Read the model definition and answer for the solid it produces. Units are mm, in the model's axes. Give positions to 0.01 mm unless a question says otherwise; leave off trailing zeros. Write each loop counter-clockwise with the first axis right and the second up, starting at its lowest first coordinate (ties: lowest second). Pieces come first, ordered by that corner, then holes. Notation, with made-up numbers: M -19.75,88.25 L 11.25,88.25 A30 cw 11.25,120.25 Z; hole C 9.5,67 d3. An arc over 180 degrees is marked long. Put each result on its own line as item: value.
Autodesk Inventor part; units mm, degrees
ref_plane "YZ Plane" through (0, 0, 0) normal (1, 0, 0) x (0, 1, 0)
ref_plane "XZ Plane" through (0, 0, 0) normal (0, 1, 0) x (-1, 0, 0)
ref_plane "XY Plane" through (0, 0, 0) normal (0, 0, 1) x (1, 0, 0)
sketch "Sketch1" plane through (0, 0, 0) normal (0, 0, 1) x (1, 0, 0)
  line L0 (-28.6, -15.9) -> (0, -15.9) construction
  line L1 (-28.6, 817.5) -> (-28.6, -17.5) construction
  line L2 (125, 817.5) -> (125, -17.5) construction
  line L3 (96.4, -15.9) -> (125, -15.9) construction
  line L4 (-28.6, 815.9) -> (0, 815.9) construction
  line L5 (96.4, 815.9) -> (125, 815.9) construction
  circle A0 centre (-14.3, 0) radius 2 construction
  circle A1 centre (110.7, 0) radius 2 construction
  circle A2 centre (-14.3, 252.5) radius 2 construction
  circle A3 centre (110.7, 252.5) radius 2 construction
  circle A4 centre (-14.3, 545.5) radius 2 construction
  circle A5 centre (110.7, 545.5) radius 2 construction
  circle A6 centre (-14.3, 800) radius 2 construction
  circle A7 centre (110.7, 800) radius 2 construction
  line L6 (-28.6, -15.9) -> (125, -15.9)
  line L7 (125, -15.9) -> (125, 815.9)
  line L8 (125, 815.9) -> (-28.6, 815.9)
  line L9 (-28.6, 815.9) -> (-28.6, -15.9)
  circle A8 centre (-14.3, 0) radius 4
  circle A9 centre (110.7, 0) radius 4
  circle A10 centre (-14.3, 252.5) radius 4
  circle A11 centre (110.7, 252.5) radius 4
  circle A12 centre (-14.3, 545.5) radius 4
  circle A13 centre (110.7, 545.5) radius 4
  circle A14 centre (-14.3, 800) radius 4
  circle A15 centre (110.7, 800) radius 4
  point P0 (0, 0)
  dimension "d0" = 2
  dimension "d1" = 2
  dimension "d2" = 2
  dimension "d3" = 2
  dimension "d4" = 2
  dimension "d5" = 2
  dimension "d6" = 2
  dimension "d7" = 2
extrude "Extrusion1" add sketch "Sketch1" along normal blind 2
sketch "Sketch2" plane through (0, 0, 2) normal (0, 0, 1) x (1, 0, 0)
  arc A0 (81.2, 144.25) -> (81.2, 152.25) centre (81.2, 148.25) ccw construction
  arc A1 (79.0077, 648.4043) -> (79.0077, 655.0957) centre (81.2, 651.75) ccw construction
  arc A2 (33.1012, 180.4907) -> (33.1012, 116.0093) centre (42.2, 148.25) ccw construction
  arc A3 (33.1012, 683.9907) -> (33.1012, 619.5093) centre (42.2, 651.75) ccw construction
  arc A4 (30.3852, 190.1148) -> (30.3852, 106.3852) centre (42.2, 148.25) ccw
  arc A5 (30.3852, 693.6148) -> (30.3852, 609.8852) centre (42.2, 651.75) ccw
  line L0 (125, -15.9) -> (125, 815.9) construction
  line L1 (30.3852, 106.3852) -> (125, 106.3852)
  line L2 (30.3852, 190.1148) -> (125, 190.1148)
  line L3 (30.3852, 609.8852) -> (125, 609.8852)
  line L4 (30.3852, 693.6148) -> (125, 693.6148)
  line L5 (125, 106.3852) -> (125, 190.1148)
  line L6 (125, 609.8852) -> (125, 693.6148)
  point P0 (0, 0)
  dimension "d10" = 10
  dimension "d11" = 10
  dimension "d16" = 83.7296
  dimension "d17" = 83.7296
  dimension "d18" = 41.8648
  dimension "d19" = 41.8648
extrude "Extrusion2" cut sketch "Sketch2" against normal blind 2
fillet "Fillet1" radius 2 8 edges at (-28.6, -15.9, 1) (125, -15.9, 1) (-28.6, 815.9, 1) (125, 815.9, 1) (125, 693.6148, 1) (125, 609.8852, 1) (125, 106.3852, 1) (125, 190.1148, 1)
sketch "Sketch3" plane through (0, 0, 2) normal (0, 0, 1) x (1, 0, 0)
  arc A0 (123, 190.1148) -> (125, 192.1148) centre (123, 192.1148) ccw construction
  line L0 (125, 192.1148) -> (125, 607.8852) construction
  arc A1 (125, 607.8852) -> (123, 609.8852) centre (123, 607.8852) ccw construction
  line L1 (123, 609.8852) -> (30.3852, 609.8852) construction
  arc A2 (30.3852, 693.6148) -> (30.3852, 609.8852) centre (42.2, 651.75) ccw construction
  line L2 (30.3852, 693.6148) -> (123, 693.6148) construction
  arc A3 (123, 693.6148) -> (125, 695.6148) centre (123, 695.6148) ccw construction
  line L3 (125, 695.6148) -> (125, 813.9) construction
  arc A4 (125, 813.9) -> (123, 815.9) centre (123, 813.9) ccw construction
  line L4 (123, 815.9) -> (-26.6, 815.9) construction
  arc A5 (-26.6, 815.9) -> (-28.6, 813.9) centre (-26.6, 813.9) ccw construction
  line L5 (-28.6, 813.9) -> (-28.6, -13.9) construction
  arc A6 (-28.6, -13.9) -> (-26.6, -15.9) centre (-26.6, -13.9) ccw construction
  line L6 (-26.6, -15.9) -> (123, -15.9) construction
  arc A7 (123, -15.9) -> (125, -13.9) centre (123, -13.9) ccw construction
  line L7 (125, -13.9) -> (125, 104.3852) construction
  arc A8 (125, 104.3852) -> (123, 106.3852) centre (123, 104.3852) ccw construction
  line L8 (123, 106.3852) -> (30.3852, 106.3852) construction
  arc A9 (30.3852, 190.1148) -> (30.3852, 106.3852) centre (42.2, 148.25) ccw construction
  line L9 (30.3852, 190.1148) -> (123, 190.1148) construction
  circle A10 centre (110.7, 800) radius 4 construction
  circle A11 centre (-14.3, 800) radius 4 construction
  circle A12 centre (110.7, 545.5) radius 4 construction
  circle A13 centre (-14.3, 545.5) radius 4 construction
  circle A14 centre (110.7, 252.5) radius 4 construction
  circle A15 centre (-14.3, 252.5) radius 4 construction
  circle A16 centre (110.7, 0) radius 4 construction
  circle A17 centre (-14.3, 0) radius 4 construction
  line L10 (-28.6, 813.9) -> (-28.6, -13.9) construction
  line L11 (-28.6, 400) -> (125, 400) construction
  line L12 (-28.6, 520) -> (125, 520) construction
  circle A18 centre (-14.3, 545.5) radius 4 construction
  line L13 (-28.6, 320) -> (125, 320) construction
  line L14 (-14.3, 545.5) -> (-14.3, 320) construction
  line L15 (110.7, 545.5) -> (110.7, 320) construction
  circle A19 centre (-14.3, 520) radius 2
  circle A20 centre (-14.3, 320) radius 2
  circle A21 centre (110.7, 320) radius 2
  circle A22 centre (110.7, 520) radius 2
  point P0 (0, 0)
  dimension "d24" = 120
  dimension "d25" = 200
  dimension "d26" = 4
  dimension "d27" = 4
  dimension "d28" = 4
  dimension "d29" = 4
extrude "Extrusion3" add sketch "Sketch3" along normal blind 10
chamfer "Chamfer1" distance 1 angle 45 4 edges at (-16.3, 320, 2) (-16.3, 520, 2) (108.7, 520, 2) (108.7, 320, 2)
thread "Thread1"
thread "Thread2"
thread "Thread3"
thread "Thread4"
sketch "Sketch4" plane through (0, 0, 2) normal (0, 0, 1) x (1, 0, 0)
  circle A0 centre (110.7, 520) radius 3 construction
  circle A1 centre (-14.3, 320) radius 3 construction
  arc A2 (123, 190.1148) -> (125, 192.1148) centre (123, 192.1148) ccw construction
  line L0 (125, 192.1148) -> (125, 607.8852) construction
  arc A3 (125, 607.8852) -> (123, 609.8852) centre (123, 607.8852) ccw construction
  line L1 (123, 609.8852) -> (30.3852, 609.8852) construction
  arc A4 (30.3852, 693.6148) -> (30.3852, 609.8852) centre (42.2, 651.75) ccw construction
  line L2 (30.3852, 693.6148) -> (123, 693.6148) construction
  arc A5 (123, 693.6148) -> (125, 695.6148) centre (123, 695.6148) ccw construction
  line L3 (125, 695.6148) -> (125, 813.9) construction
  arc A6 (125, 813.9) -> (123, 815.9) centre (123, 813.9) ccw construction
  line L4 (123, 815.9) -> (-26.6, 815.9) construction
  arc A7 (-26.6, 815.9) -> (-28.6, 813.9) centre (-26.6, 813.9) ccw construction
  line L5 (-28.6, 813.9) -> (-28.6, -13.9) construction
  arc A8 (-28.6, -13.9) -> (-26.6, -15.9) centre (-26.6, -13.9) ccw construction
  line L6 (-26.6, -15.9) -> (123, -15.9) construction
  arc A9 (123, -15.9) -> (125, -13.9) centre (123, -13.9) ccw construction
  line L7 (125, -13.9) -> (125, 104.3852) construction
  arc A10 (125, 104.3852) -> (123, 106.3852) centre (123, 104.3852) ccw construction
  line L8 (123, 106.3852) -> (30.3852, 106.3852) construction
  arc A11 (30.3852, 190.1148) -> (30.3852, 106.3852) centre (42.2, 148.25) ccw construction
  line L9 (30.3852, 190.1148) -> (123, 190.1148) construction
  circle A12 centre (110.7, 800) radius 4 construction
  circle A13 centre (-14.3, 800) radius 4 construction
  circle A14 centre (110.7, 545.5) radius 4 construction
  circle A15 centre (-14.3, 545.5) radius 4 construction
  circle A16 centre (110.7, 252.5) radius 4 construction
  circle A17 centre (-14.3, 252.5) radius 4 construction
  circle A18 centre (110.7, 0) radius 4 construction
  circle A19 centre (-14.3, 0) radius 4 construction
  circle A20 centre (-14.3, 520) radius 3 construction
  circle A21 centre (110.7, 320) radius 3 construction
  circle A22 centre (-14.3, 320) radius 2 construction
  circle A23 centre (110.7, 252.5) radius 4 construction
  line L10 (110.7, 252.5) -> (-14.3, 252.5) construction
  line L11 (-14.3, 252.5) -> (-14.3, 320) construction
  line L12 (-14.3, 320) -> (110.7, 320) construction
  line L13 (110.7, 320) -> (110.7, 252.5) construction
  line L14 (48.2, 252.5) -> (48.2, 320) construction
  line L15 (0.7, 267.5) -> (95.7, 267.5) construction
  line L16 (95.7, 267.5) -> (95.7, 305) construction
  line L17 (95.7, 305) -> (0.7, 305) construction
  line L18 (0.7, 305) -> (0.7, 267.5) construction
  line L19 (2.7, 267.5) -> (46.2, 267.5)
  line L20 (48.2, 269.5) -> (48.2, 303)
  line L21 (46.2, 305) -> (2.7, 305)
  line L22 (0.7, 303) -> (0.7, 269.5)
  arc A24 (0.7, 269.5) -> (2.7, 267.5) centre (2.7, 269.5) ccw
  arc A25 (2.7, 305) -> (0.7, 303) centre (2.7, 303) ccw
  arc A26 (46.2, 267.5) -> (48.2, 269.5) centre (46.2, 269.5) ccw
  arc A27 (48.2, 303) -> (46.2, 305) centre (46.2, 303) ccw
  point P0 (0, 0)
  point P1 (48.2, 305)
  dimension "d43" = 15
  dimension "d44" = 2
  dimension "d45" = 2
  dimension "d46" = 2
  dimension "d47" = 2
extrude "Extrusion4" cut sketch "Sketch4" against normal up to next
properties part number "Cover_Left"
(1) Section B-B on z = 6 is taken. Determine the outline of the cut face in (x, y), and give its area (3 significant figures).
Result:
outline: C -14.3,320 d4; C -14.3,520 d4; C 110.7,320 d4; C 110.7,520 d4
area: 50.3 mm²
(2) Section A-A on x = 61.5 is taken. Determine the outline of the cut face in (y, z), and give its area (3 significant figures).
Result:
outline: M -15.9,0 L 106.39,0 L 106.39,2 L -15.9,2 Z; M 190.11,0 L 609.89,0 L 609.89,2 L 190.11,2 Z; M 693.61,0 L 815.9,0 L 815.9,2 L 693.61,2 Z
area: 1,330 mm²
(3) Section C-C on x = 16 is taken. Determine the outline of the cut face in (y, z), and give its area (3 significant figures).
Result:
outline: M -15.9,0 L 113.53,0 L 113.53,2 L -15.9,2 Z; M 182.97,0 L 267.5,0 L 267.5,2 L 182.97,2 Z; M 305,0 L 617.03,0 L 617.03,2 L 305,2 Z; M 686.47,0 L 815.9,0 L 815.9,2 L 686.47,2 Z
area: 1,310 mm²
(4) Section D-D on y = 97.5 is taken. Determine the outline of the cut face in (x, z), and give its area (3 significant figures).
Result:
outline: M -28.6,0 L 125,0 L 125,2 L -28.6,2 Z
area: 307 mm²
(5) Straight lines are drawn through the part: line 1 along X through (y, z) = (545.5, 0.85); line 2 along Y through (x, z) = (-14.3, 1.55); line 3 along Y through (x, z) = (74, 1.75). For each, find the intervals that lie inside material, in ascending order. Write a range as from..to.
Result:
line 1: x = -28.6..-18.3, -10.3..106.7, 114.7..125
line 2: y = -15.9..-4, 4..248.5, 256.5..541.5, 549.5..796, 804..815.9
line 3: y = -15.9..106.39, 190.11..609.89, 693.61..815.9
(6) Given pin 1 Ø1 at (x, y) = (44.5, 706.5) entering from +Z, flat-ended and moving along its own axis, determine where the tip first touches the part or whether it passes through.
Result:
pin 1: stops at z = 2
(7) For a pull along Y with two mould halves and no side action, classify faces 1 (the face through (47, 406, 0)), 2 (the face through (-1.293, 149.039, 1.014)) as +Y half, -Y half, draft (parallel to the pull), parting line (faces both ways), or undercut.
Result:
face 1: draft
face 2: undercut
